Input: part model. Units: mm. Frame: model coordinates. A direction names the side the tool comes from. Round coordinates to 2 decimals unless told otherwise and drop trailing zeros. Loops run counter-clockwise (first coordinate to the right, second up) from the corner with the lowest first, then second, coordinate; pieces in that order, holes last. Notation, with made-up numbers: M 33.25,81.5 L 48.25,81.5 A19 ccw 48.25,116.5 Z; hole C -30.5,-3 d9. An arc over 180 degrees is marked long. Put each result on its own line as item: value. Start each with the question number.
1) Section C-C on y = -131. Output: boundary loops of the cut face in (x, z), plus the area to 3 significant figures.
2) Section B-B on z = -55. Output: boundary loops of the cut face in (x, y), plus the area to 3 significant figures.
3) Section A-A on x = -160. Output: boundary loops of the cut face in (y, z).
4) Section D-D on x = -123. Output: boundary loops of the cut face in (y, z), plus the area to 3 significant figures.
5) Line query: probe 1 along X at (y, z) = (-108, -59.5); probe 2 along Y at (x, z) = (-81, -29.5); probe 3 along Y at (x, z) = (-71.5, -47.5). Output: solid intervals per line, ascending.
6) Pin query (flat end, axial travel): pin 1 (5 mm diameter, centred on y = -41, z = 28.5, fed in from -X); pin 2 (12 mm diameter, centred on x = -43, z = -22.5, fed in from -Y); pin 3 (3 mm diameter, centred on x = -33, z = 39, fed in from +Y); pin 4 (5.5 mm diameter, centred on x = -150.8, y = -116.4, fed in from +Z). Return the tip coordinate at first contact, or that it passes through.
7) Reachability of faces 1 (the face through (-107.06, -152.9, 74.34)), 2 (the face through (-151.07, -137.79, 74.34)), 3 (the face through (26.298, -175.222, -1.085)), 4 (the face through (-138, -126, -71.12)), 5 (the face through (-161.472, -93.226, 74.339)) from +Z, -Z, +X, -X, +Y, -Y: full face, straight path, thin tool, end or side. Return the list, or none.
8) Draft query along Z for faces 6 (the face through (-161.472, -93.226, -74.339)), 7 (the face through (-125.22, -128.01, 1.08)), 8 (the face through (-122, -129, 77.47)), 9 (the face through (-138, -126, 71.12)). Return one class per face: +Z half, -Z half, draft (parallel to the pull), parting line (faces both ways), or undercut.
from build123d import *

# Parameters (mm, degrees)
BOSS_EXTRUDE1_DEPTH = 77.47
BOSS_EXTRUDE2_DEPTH = 6.35
SKETCH3_R           = 2.3495
CUT_EXTRUDE2_DEPTH  = 297.881345658
CHAMFER1_START      = -172.258951726
CHAMFER1_OUTLINE_W  = 62
CHAMFER1_OUTLINE_H  = 158
CHAMFER1_DEPTH      = 6.258951726


with BuildPart() as part:
    # Sketch1 → Boss-Extrude1 (new, symmetric)
    with BuildSketch(Plane.XY):
        with BuildLine():
            Line((-179.07, 0), (-172.72, 0))
            ThreePointArc((-172.72, 0), (-122.131483247, -122.131483247), (0, -172.72))
            Line((0, -172.72), (55.88, -172.72))
            Line((55.88, -172.72), (55.88, -179.07))
            Line((55.88, -179.07), (0, -179.07))
            ThreePointArc((0, -179.07), (-126.621611307, -126.621611307), (-179.07, 0))
        make_face()
    extrude(amount=BOSS_EXTRUDE1_DEPTH, both=True)

    # Sketch2 → Boss-Extrude2 (add)
    with BuildSketch(Plane.XY.offset(77.47)):
        with BuildLine():
            Line((-155.079169056, -89.535), (-168.047204306, -97.022098643))
            ThreePointArc((-168.047204306, -97.022098643), (-172.846425248, -103.448872568), (-171.488365315, -111.354036575))
            ThreePointArc((-171.488365315, -111.354036575), (-150.751097058, -138.137929751), (-125.876496699, -161.130656546))
            ThreePointArc((-125.876496699, -161.130656546), (-118.11977695, -163.172529091), (-111.299179173, -158.951700888))
            Line((-111.299179173, -158.951700888), (-102.710332457, -146.685556571))
            ThreePointArc((-102.710332457, -146.685556571), (-132.024252703, -120.977938478), (-155.079169056, -89.535))
        make_face()
    boss_extrude2 = extrude(amount=-BOSS_EXTRUDE2_DEPTH)

    # Mirror1: Boss-Extrude2 across plane
    add(boss_extrude2.mirror(Plane.XY))

    # Sketch3 → Cut-Extrude2 (cut, through all)
    with BuildSketch(Plane.XY.offset(77.47)):
        with Locations((-150.804793508, -116.396581802)):
            Circle(SKETCH3_R)
        with Locations((-129.097161455, -140.086305199)):
            Circle(SKETCH3_R)
    extrude(amount=-CUT_EXTRUDE2_DEPTH, mode=Mode.SUBTRACT)

    # Chamfer1: read off the stored shape, not the designer's step
    # Chamfer1 outline → Chamfer1 (cut)
    with BuildSketch(Plane(origin=(0, 0, 0), x_dir=(0.996185998135626, -0.0872551266031199, 0), z_dir=(0.0872551266031199, 0.996185998135626, 0)).offset(CHAMFER1_START)):
        with Locations((42, 0)):
            Rectangle(CHAMFER1_OUTLINE_W, CHAMFER1_OUTLINE_H)
    extrude(amount=CHAMFER1_DEPTH, mode=Mode.SUBTRACT)


solid = part.part
Geometry results:
1. outline: M -156.99,-77.47 L -112.57,-77.47 L -112.57,77.47 L -156.99,77.47 L -156.99,71.12 L -122.09,71.12 L -122.09,-71.12 L -156.99,-71.12 Z
1. area: 1,920 mm²
2. outline: M -179.07,0 A179.07 ccw 0,-179.07 L 55.88,-179.07 L 55.88,-177.81 L -2.47,-172.7 A172.72 cw -172.72,0 Z
2. area: 1,960 mm²
3. outline: M -127.31,-77.47 L -92.38,-77.47 L -92.38,-71.12 L -127.31,-71.12 Z; M -127.31,71.12 L -92.38,71.12 L -92.38,77.47 L -127.31,77.47 Z; M -80.41,-77.47 L -65.06,-77.47 L -65.06,77.47 L -80.41,77.47 Z
4. outline: M -162.71,-77.47 L -121.26,-77.47 L -121.26,77.47 L -162.71,77.47 L -162.71,71.12 L -130.14,71.12 L -130.14,-71.12 L -162.71,-71.12 Z
4. area: 1,790 mm²
5. probe 1: x = -142.84 to -134.79
5. probe 2: y = -159.7 to -152.55
5. probe 3: y = -164.18 to -157.23
6. pin 1: stops at x = -174.88
6. pin 2: stops at y = -175.21
6. pin 3: stops at y = -169.24
6. pin 4: stops at z = 77.47
7. face 1: +Z, -Z, -Y
7. face 2: +Z, -Z, -X, -Y
7. face 3: +Z, -Z, +X, +Y
7. face 4: -X, -Y
7. face 5: +Z, -Z, -X
8. face 6: draft
8. face 7: undercut
8. face 8: +Z half
8. face 9: undercut
